Source: CAD feature listing. Evaluate the final solid. Frame: model axes, mm. Give positions to 0.01 mm unless a question says otherwise; leave off trailing zeros. Order: outer loops, then holes, each group sorted by start corner. A loop starts at its lowest first (then second) coordinate and runs counter-clockwise, first axis right, second up. Notation, with made-up numbers: M -36.75,-11.75 L -14.75,-11.75 A9 ccw -14.75,-7.75 Z; hole C -10.75,14 d3. An arc over 180 degrees is marked long. Use CSV: the item, a comma, the result in double quotes. Start each with the question number.
Item 1: Section query B-B on y = -50. Return loops of the section in (x, z) (3 decimals).
Item 2: Pull-direction query (X, two-part tool) for faces 1 (the face through (3.336, -34.976, 3.042)), 2 (the face through (-3, 3, 6)); classes: +X half, -X half, draft (parallel to the pull), parting line (faces both ways), or undercut.
Item 3: First-contact query: pin 1 (3 mm diameter, centred on x = -117.5, y = 74, fed in from -Z). Flat tip, straight axial feed; report the tip coordinate or a pass-through.
Item 4: Section query A-A on x = 0. Return loops of the section in (y, z) (3 decimals).
Item 5: Ray query, probe 1 along Y at (x, z) = (0, 2) (3 decimals); probe 2 along X at (y, z) = (-50, 1.4) (3 decimals); probe 3 along X at (y, z) = (-57, 2.1) (3 decimals). Return the intervals inside material, ascending. Write a range as from..to.
from build123d import *

# Parameters (mm, degrees)
SKETCH_W              = 399.99
SKETCH_H              = 399.99
PAD_DEPTH             = 6
SKETCH001_R           = 15.39
POCKET_DEPTH          = 1137.407205
POLARPATTERN001_COUNT = 2


with BuildPart() as part:
    # Sketch → Pad (new body)
    with BuildSketch(Plane.XY):
        Rectangle(SKETCH_W, SKETCH_H)
    extrude(amount=PAD_DEPTH)

    # Sketch001 (on Face6 of Pad) → Pocket (cut, through all)
    with BuildSketch(Plane.XY.offset(6)):
        with Locations((0, 50)):
            Circle(SKETCH001_R)
    pocket = extrude(amount=-POCKET_DEPTH, mode=Mode.SUBTRACT)

    # PolarPattern001: Pocket ×2 about axis
    polarpattern001_axis = Axis((0, 0, 6), (0, 0, 1))
    for i in range(1, POLARPATTERN001_COUNT):
        add(pocket.rotate(polarpattern001_axis, i * 360 / POLARPATTERN001_COUNT), mode=Mode.SUBTRACT)


solid = part.part
Verdict:
1,outline,"M -199.995,0 L -15.39,0 L -15.39,6 L -199.995,6 Z; M 15.39,0 L 199.995,0 L 199.995,6 L 15.39,6 Z"
2,face 1,"undercut"
2,face 2,"draft"
3,pin 1,"z = 0"
4,outline,"M -199.995,0 L -65.39,0 L -65.39,6 L -199.995,6 Z; M -34.61,0 L 34.61,0 L 34.61,6 L -34.61,6 Z; M 65.39,0 L 199.995,0 L 199.995,6 L 65.39,6 Z"
5,probe 1,"-199.995..-65.39, -34.61..34.61, 65.39..199.995"
5,probe 2,"-199.995..-15.39, 15.39..199.995"
5,probe 3,"-199.995..-13.706, 13.706..199.995"
